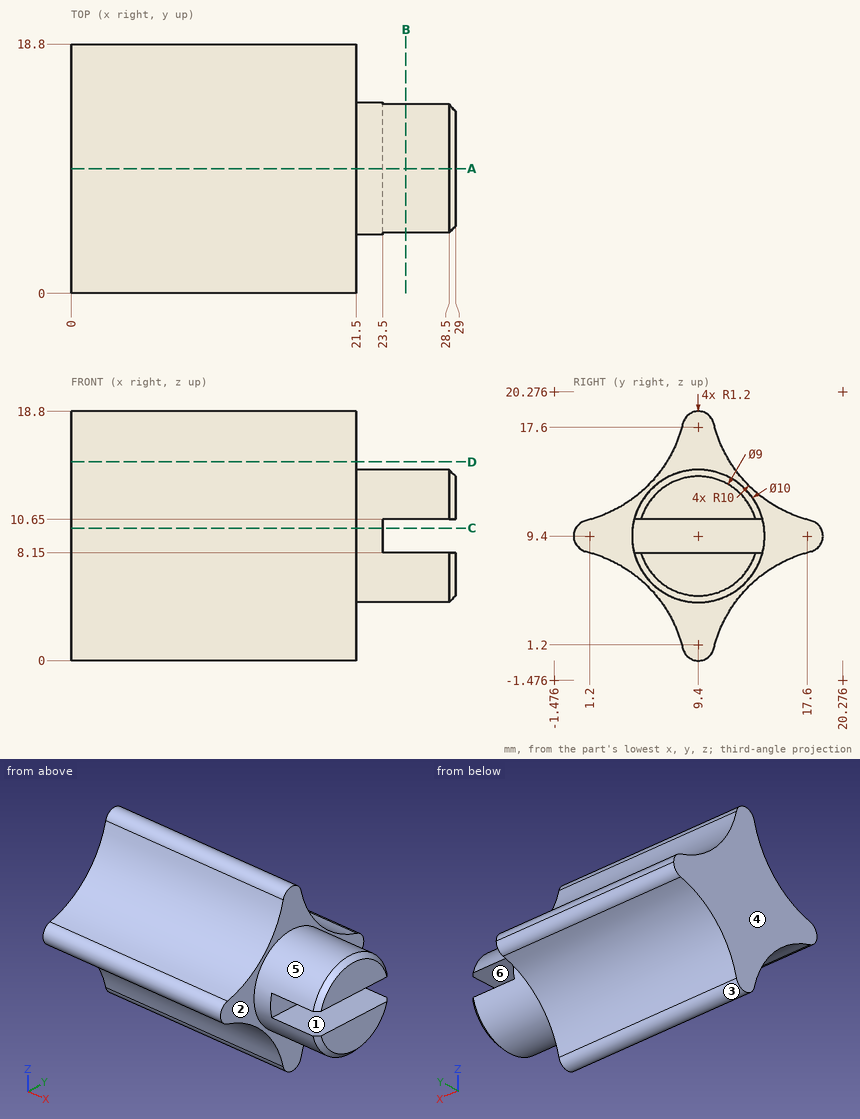
Design review of the part shown in the three views and the two pictorial views. Dimensions are in mm from the part's minimum x, y and z. A direction names the side the tool comes from. Give positions to 0.01 mm unless a question says otherwise; leave off trailing zeros. Write each loop counter-clockwise with the first axis right and the second up, starting at its lowest first coordinate (ties: lowest second). Pieces come first, ordered by that corner, then holes.
(1) Wall thickness on line 1 along X through (y, z) = (16.75, 8.25); line 2 along Z through (x, y) = (23.75, 11.75); line 3 along X through (y, z) = (8.25, 8.5): over which ranges is each line inside the solid? List them lowest first.
Checked values:
line 1: x = 0 to 21.5
line 2: z = 4.99 to 8.15, 10.65 to 13.81
line 3: x = 0 to 23.5
(2) Add section D-D (z = 15). Give the boundary of the cut face in (x, y), and give its area (3 significant figures).
Checked values:
outline: (0, 7.02) - (21.5, 7.02) - (21.5, 11.78) - (0, 11.78) - close
area: 102 mm2
(3) Add section B-B (x = 25.25). Give the boundary of the cut face in (y, z), and give its area (3 significant figures).
Checked values:
outline: (4.56, 8.15) arc R5 ccw to (14.24, 8.15) - close; (4.56, 10.65) - (14.24, 10.65) arc R5 ccw to start
area: 53.8 mm2
(4) Clearance check with flat-ended pins moving along their axes: pin 1 Ø4.5 at (x, y) = (26.5, 10) entering from -Z; pin 2 Ø0.8 at (y, z) = (7.5, 10) entering from +X; pin 3 Ø1.6 at (x, y) = (27, 9) entering from +Z. State where each tip first meets the part, or that it passes through.
Checked values:
pin 1: stops at z = 4.4
pin 2: stops at x = 23.5
pin 3: stops at z = 14.4
(5) Add section C-C (z = 10). Give the boundary of the cut face in (x, y), and give its area (3 significant figures).
Checked values:
outline: (0, 0.16) - (21.5, 0.16) - (21.5, 4.44) - (23.5, 4.44) - (23.5, 14.36) - (21.5, 14.36) - (21.5, 18.64) - (0, 18.64) - close
area: 417 mm2
(6) Add section A-A (y = 9.4). Give the boundary of the cut face in (x, z).
Checked values:
outline: (0, 0) - (21.5, 0) - (21.5, 4.4) - (28.5, 4.4) - (29, 4.9) - (29, 8.15) - (23.5, 8.15) - (23.5, 10.65) - (29, 10.65) - (29, 13.9) - (28.5, 14.4) - (21.5, 14.4) - (21.5, 18.8) - (0, 18.8) - close
(7) Mouldability with a two-part tool opening along Z and no side actions: class the marked faces 4, 5 and 6 as +Z half, -Z half, draft (parallel to the pull), parting line (faces both ways), or undercut.
Checked values:
face 4: draft
face 5: parting line
face 6: undercut
(8) Tool access review of the marked faces 1, 2 and 3: name each direction out of +Z, -Z, +X, -X, +Y, -Y from which nothing blocks a thin tool from reaching the whole face with its end or side.
Checked values:
face 1: +X, +Y, -Y
face 2: +X
face 3: -Z, +X, -X
